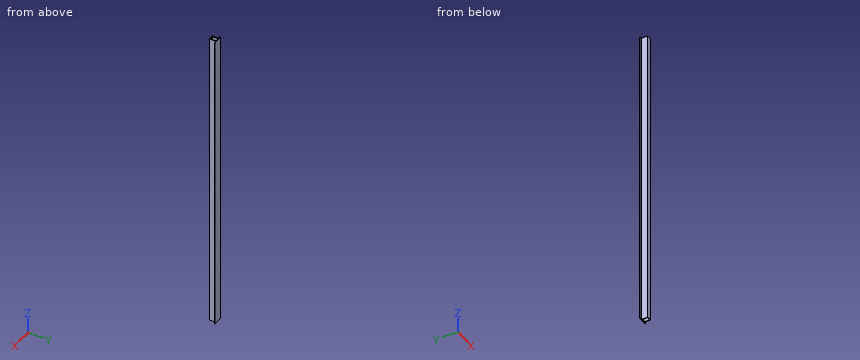
Autodesk Inventor part; units mm, degrees
ref_plane "YZ Plane" through (0, 0, 0) normal (1, 0, 0) x (0, 1, 0)
ref_plane "XZ Plane" through (0, 0, 0) normal (0, 1, 0) x (-1, 0, 0)
ref_plane "XY Plane" through (0, 0, 0) normal (0, 0, 1) x (1, 0, 0)
sketch "Skizze1" plane through (0, 0, 0) normal (0, 0, 1) x (1, 0, 0)
  line L0 (0, 0) -> (30, 0)
  line L1 (30, 0) -> (30, -2)
  line L2 (30, -2) -> (0, -2)
  line L3 (0, -2) -> (0, 0)
  line L4 (7.5, -2) -> (9.5, -2)
  line L5 (9.5, -2) -> (9.5, -22)
  line L6 (9.5, -22) -> (7.5, -22)
  line L7 (7.5, -22) -> (7.5, -2)
  line L8 (9.5, -22) -> (20.5, -22)
  line L9 (20.5, -22) -> (20.5, -20)
  line L10 (20.5, -20) -> (9.5, -20)
  line L11 (9.5, -20) -> (9.5, -22)
  line L12 (20.5, -22) -> (22.5, -22)
  line L13 (22.5, -22) -> (22.5, -2)
  line L14 (22.5, -2) -> (20.5, -2)
  line L15 (20.5, -2) -> (20.5, -22)
  line L16 (15, -20) -> (15, -2) construction
  point P0 (20.5, -2)
  point P1 (9.5, -2)
  dimension "d0" = 30
  dimension "d1" = 2
  dimension "d2" = 2
  dimension "d3" = 20
  dimension "d4" = 11
  dimension "d5" = 2
  dimension "d6" = 2
  dimension "d7" = 7.5
  dimension "d8" = 20.5
  dimension "d9" = 20
  dimension "d12" = 7.5
extrude "Extrusion1" add sketch "Skizze1" along normal blind 1000 contours L0 L1 L2 L3 | L2 L5 L6 L7 | L13 L12 L9 L15 L2 | L10 L9 L8 L5
properties part number "TrägerUI" material "Aluminium 6061, Katze"
CAD build for the part. Positions are in the model's coordinates, mm. Round coordinates to 2 decimals unless told otherwise and drop trailing zeros. Loops run counter-clockwise (first coordinate to the right, second up) from the corner with the lowest first, then second, coordinate; pieces in that order, holes last.
(1) Cut at B-B (y = -14.75). Give the cut face in (x, z).
(2) Wall check: line 1 along X through (y, z) = (-18, 898); line 2 along Y through (x, z) = (18.5, 480); line 3 along Y through (x, z) = (23.25, 493.5). Give the ranges that are in metal, low to high.
(3) Cut at A-A (z = 350). Give the cut face in (x, y), plus the area to 3 significant figures.
(4) Drop flat-ended pins along their axis: pin 1 (5.5 mm diameter, centred on y = -6.5, z = 562, fed in from +X); pin 2 (10 mm diameter, centred on x = 4, z = 727.5, fed in from -Y); pin 3 (4 mm diameter, centred on x = 2, z = 599.5, fed in from -Y); pin 4 (1.5 mm diameter, centred on x = 6.5, y = -12, fed in from +Z). Give the stop position or say it passes through.
Findings below:
1. outline: (7.5, 0) - (9.5, 0) - (9.5, 1000) - (7.5, 1000) - close; (20.5, 0) - (22.5, 0) - (22.5, 1000) - (20.5, 1000) - close
2. line 1: x = 7.5 to 9.5, 20.5 to 22.5
2. line 2: y = -22 to -20, -2 to 0
2. line 3: y = -2 to 0
3. outline: (0, -2) - (7.5, -2) - (7.5, -22) - (22.5, -22) - (22.5, -2) - (30, -2) - (30, 0) - (0, 0) - close; hole (9.5, -20) - (20.5, -20) - (20.5, -2) - (9.5, -2) - close
3. area: 162 mm2
4. pin 1: stops at x = 22.5
4. pin 2: stops at y = -22
4. pin 3: stops at y = -2
4. pin 4: passes through
